```python
from build123d import *

# Parameters (mm, degrees)
EXTRUDE1_DEPTH           = 0.889
SKETCH2_R                = 2.0828
EXTRUDE2_DEPTH           = 144.686848114
CHAMFER1_SIZE            = 0.889
CHAMFER1_OF_MIRROR1_SIZE = 0.889


with BuildPart() as part:
    # Sketch1 → Extrude1 (new, symmetric)
    with BuildSketch(Plane.XY):
        Polygon((0, 101.6), (0, 0), (101.6, 0), (101.6, 15.875), (15.875, 15.875), (15.875, 101.6), align=None)
    extrude(amount=EXTRUDE1_DEPTH, both=True)

    # Sketch2 → Extrude2 (cut, symmetric)
    with BuildSketch(Plane.XY):
        with Locations((-14.224, 7.9375)):
            Circle(SKETCH2_R)
        with Locations((36.576, 7.9375)):
            Circle(SKETCH2_R)
        with Locations((81.026, 7.9375)):
            Circle(SKETCH2_R)
    extrude2 = extrude(amount=EXTRUDE2_DEPTH, both=True, mode=Mode.SUBTRACT)

    # Chamfer1
    chamfer1_edges = [part.edges().sort_by_distance(p)[0] for p in [
        (34.4932, 7.9375, 0.889),
        (78.9432, 7.9375, 0.889),
    ]]
    chamfer(chamfer1_edges, length=CHAMFER1_SIZE)

    # Mirror1: Extrude2 across plane
    add(extrude2.mirror(Plane(origin=(0, 0, 0), x_dir=(0, 0, 1), z_dir=(-0.7071067811865477, 0.7071067811865474, 0))), mode=Mode.SUBTRACT)

    # Chamfer1 of Mirror1
    chamfer1_of_mirror1_edges = [part.edges().sort_by_distance(p)[0] for p in [
        (7.9375, 34.4932, 0.889),
        (7.9375, 78.9432, 0.889),
    ]]
    chamfer(chamfer1_of_mirror1_edges, length=CHAMFER1_OF_MIRROR1_SIZE)


solid = part.part
```
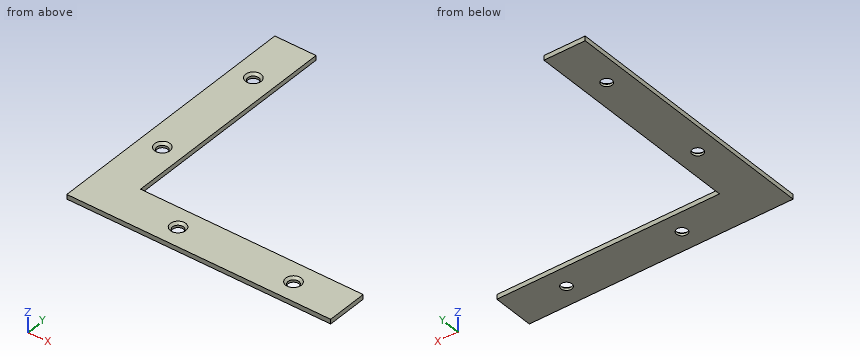
Input: part model. Units: mm. Frame: model coordinates. Round coordinates to 2 decimals unless told otherwise and drop trailing zeros. Write each loop counter-clockwise with the first axis right and the second up, starting at its lowest first coordinate (ties: lowest second). Pieces come first, ordered by that corner, then holes. Notation, with made-up numbers: (19, 89.25) -> (77, 89.25) arc R14 cw to (77, 94.25) -> close; hole circle Ø8 at (-26.5, 28). An arc over 180 degrees is marked (long way). Answer as CSV lines item,"result".
1. Ray query, L1, parallel to X at y = 45, z = 0.1 (3 decimals); L2, parallel to X at y = 82.5, z = -0.6 (3 decimals). Return the intervals inside material, ascending. Write a range as [from, to].
Geometry says:
L1,"x = [0, 15.875]"
L2,"x = [0, 6.466], [9.409, 15.875]"
2. Contact query for flat-ended pins moving along their axis: P1, Ø3.5, axis at x = 81.03, y = 7.94, coming from the +Z side; P2, Ø0.5, axis at y = 39, z = 0, coming from the +X side (3 decimals). Output: stop coordinate, or through.
Geometry says:
P1,"passes through"
P2,"stops at x = 15.875"
3. Section B-B (x = 41). Return the cut outline in (y, z) (3 decimals), plus the area to 3 significant figures.
Geometry says:
outline,"(0, -0.889) -> (15.875, -0.889) -> (15.875, 0.889) -> (0, 0.889) -> close"
area,"28.2 mm^2"
4. Section A-A (z = -0.35). Return the cut outline in (x, y) (1 decimal), plus the area to 3 significant figures.
Geometry says:
outline,"(0, 0) -> (101.6, 0) -> (101.6, 15.9) -> (15.9, 15.9) -> (15.9, 101.6) -> (0, 101.6) -> close; hole circle Ø4.2 at (7.9, 36.6); hole circle Ø4.2 at (7.9, 81); hole circle Ø4.2 at (36.6, 7.9); hole circle Ø4.2 at (81, 7.9)"
area,"2,920 mm^2"
